```python
from build123d import *

# Parameters (mm, degrees)
SKETCH2_R           = 5
BOSS_EXTRUDE1_DEPTH = 10
FILLET1_R           = 3
SKETCH3_R           = 5
BOSS_EXTRUDE2_DEPTH = 10
SKETCH4_R           = 6
SKETCH4_R_2         = 4.5
BOSS_EXTRUDE3_DEPTH = 2
SKETCH6_R           = 4.5
BOSS_EXTRUDE4_DEPTH = 12


with BuildPart() as part:
    # Sketch2 → Boss-Extrude1 (new body)
    with BuildSketch(Plane(origin=(0, 0, 0), x_dir=(1, 0, 0), z_dir=(0, 1, 0))):
        with BuildLine():
            ThreePointArc((-8.065392234, -5.911805826), (5.911805826, -8.065392234), (8.065392234, 5.911805826))
            ThreePointArc((8.065392234, 5.911805826), (-47.75, 34.203568305), (-103.565392234, 5.911805826))
            ThreePointArc((-103.565392234, 5.911805826), (-101.411805826, -8.065392234), (-87.434607766, -5.911805826))
            ThreePointArc((-87.434607766, -5.911805826), (-47.75, 14.203568305), (-8.065392234, -5.911805826))
        make_face()
        with Locations((-95.5, 0)):
            Circle(SKETCH2_R, mode=Mode.SUBTRACT)
        Circle(SKETCH2_R, mode=Mode.SUBTRACT)
    extrude(amount=BOSS_EXTRUDE1_DEPTH)

    # Fillet1
    fillet1_edges = [part.edges().sort_by_distance(p)[0] for p in [
        (5.911805826, 10, 8.065392234),
        (-47.75, 10, -34.203568305),
        (-101.411805826, 10, 8.065392234),
        (-47.75, 10, -14.203568305),
        (-47.75, 0, -14.203568305),
        (-101.411805826, 0, 8.065392234),
        (-47.75, 0, -34.203568305),
        (5.911805826, 0, 8.065392234),
    ]]
    fillet(fillet1_edges, radius=FILLET1_R)

    # Sketch3 → Boss-Extrude2 (add)
    with BuildSketch(Plane(origin=(0, 10, 0), x_dir=(1, 0, 0), z_dir=(0, 1, 0))):
        Circle(SKETCH3_R)
    extrude(amount=-BOSS_EXTRUDE2_DEPTH)

    # Sketch4 → Boss-Extrude3 (add)
    with BuildSketch(Plane(origin=(0, 10, 0), x_dir=(1, 0, 0), z_dir=(0, 1, 0))):
        Circle(SKETCH4_R)
        Circle(SKETCH4_R_2, mode=Mode.SUBTRACT)
    extrude(amount=BOSS_EXTRUDE3_DEPTH)

    # Sketch6 → Boss-Extrude4 (add)
    with BuildSketch(Plane(origin=(0, 10, 0), x_dir=(1, 0, 0), z_dir=(0, 1, 0))):
        Circle(SKETCH6_R)
    extrude(amount=BOSS_EXTRUDE4_DEPTH)


solid = part.part
```
Geometry check sheet. Reference: the model listing, model coordinates, mm. A direction names the side the tool comes from. Round coordinates to 2 decimals unless told otherwise and drop trailing zeros. Order: outer loops, then holes, each group sorted by start corner. A loop starts at its lowest first (then second) coordinate and runs counter-clockwise, first axis right, second up. Notation, with made-up numbers: (33, -27.75) -> (54, -27.75) arc R25 ccw to (54, 2.25) -> close; hole circle Ø3 at (-1, 9). An arc over 180 degrees is marked (long way). Return JSON: item names as keys, results as strings. Group by question number.
Q1. Release check for a two-part mould opening along X. For faces 1 (the flat face through (-52, 10, -18)), 2 (the cylindrical face through (-48.4, 5, -14.2)), 3 (the cylindrical face through (-46.841, 4.972, -34.198)) record: released by +X, released by -X, zero draft, split by the parting line, or undercut.
Q2. Tool access check on faces 4 (the flat face through (-1.4, 12, -4.5)), 5 (the cylindrical face through (-90.881, 4.93, 1.915)). Record the directions out of +Z, -Z, +X, -X, +Y, -Y that give a thin tool (end or side, any length) a straight path to the whole face; none if there is none.
Q3. Gauge pin test, flat ends, axial feed: pin 1 (1.5 mm diameter, centred on y = 12.5, z = -1.5, fed in from +X); pin 2 (4 mm diameter, centred on x = -83.5, y = 8, fed in from -Z); pin 3 (5 mm diameter, centred on x = -15, z = -26, fed in from +Y); pin 4 (8 mm diameter, centred on x = -95.5, z = 0, fed in from +Y). Record the tip position at first contact, or that the pin passes through.
Q4. Section check C-C, the plane y = 13.5. Record the boundary of the cut face in (x, z), plus the area to 3 significant figures.
Q5. Section check B-B, the plane z = 0. Count the separate pieces of the cut face and the enclosed holes in it, plus the area to 3 significant figures.
Q6. Material ranges on probe 1 along X at (y, z) = (6.25, 0); probe 2 along Z at (x, y) = (-95.5, 4.5); probe 3 along X at (y, z) = (2, -4), recorded low to high. Write a range as from..to.
Numbers:
{
 "1": {"face 1": "zero draft", "face 2": "undercut", "face 3": "split by the parting line"},
 "2": {"face 4": "+Y", "face 5": "+Y, -Y"},
 "3": {"pin 1": "x = 5.93", "pin 2": "z = -25.33", "pin 3": "y = 9.95", "pin 4": "through"},
 "4": {"outline": "circle Ø9 at (0, 0)", "area": "63.6 mm^2"},
 "5": {"separate pieces": "3", "enclosed holes": "0", "area": "459 mm^2"},
 "6": {"probe 1": "-105.5..-100.5, -90.5..-82.33, -13.17..10", "probe 2": "-15.09..-5, 5..10", "probe 3": "-104.48..-98.5, -92.5..-78.03, -17.47..8.98"}
}
